from build123d import *

# Parameters (mm, degrees)
F0_R     = 2.1
F1_DEPTH = 6.16
F2_W     = 23
F2_H     = 3
F3_DEPTH = 12.5
F4_W     = 23
F4_H     = 20
F4_W_2   = 2.2
F4_H_2   = 1.7
F5_DEPTH = 1.6
F8_DEPTH = 2
F12_R    = 2


with BuildPart() as f1:
    # F0 (on Right) → F1 (new body)
    with BuildSketch(Plane.YZ):
        Polygon((-9.7124977037, -5.25), (9.7124977037, -5.25), (11.5, -3.4624977037), (11.5, 3.4624977037), (11.5, 5.25), (9.7124977037, 5.25), (-9.7124977037, 5.25), (-11.5, 5.25), (-11.5, 3.4624977037), (-11.5, -3.4624977037), align=None)
        with Locations((-6.35, 0)):
            Circle(F0_R, mode=Mode.SUBTRACT)
        with Locations((6.35, 0)):
            Circle(F0_R, mode=Mode.SUBTRACT)
    extrude(amount=F1_DEPTH)

    # F2 (on face) → F3 (join)
    with BuildSketch(Plane(origin=(0, 0, 0), x_dir=(0, -1, 0), z_dir=(-1, 0, 0))):
        with Locations((0, 6.75)):
            Rectangle(F2_W, F2_H)
    extrude(amount=-F3_DEPTH)

    # F4 (on face) → F5 (join)
    with BuildSketch(Plane.YZ.offset(12.5)):
        with Locations((0, 15.25)):
            Rectangle(F4_W, F4_H)
        with Locations((-2.65, 9.4)):
            Rectangle(F4_W_2, F4_H_2, mode=Mode.SUBTRACT)
        with Locations((2.65, 9.4)):
            Rectangle(F4_W_2, F4_H_2, mode=Mode.SUBTRACT)
        with Locations((-2.65, 23.1)):
            Rectangle(F4_W_2, F4_H_2, mode=Mode.SUBTRACT)
        with Locations((2.65, 23.1)):
            Rectangle(F4_W_2, F4_H_2, mode=Mode.SUBTRACT)
    extrude(amount=-F5_DEPTH)

    # F6: union 

    # F7 (on face) → F8 (join)
    with BuildSketch(Plane(origin=(0, 11.5, 0), x_dir=(-1, 0, 0), z_dir=(0, 1, 0))):
        Polygon((-5.45, 8.25), (-10.9, 14.6002341062), (-10.9, 8.25), align=None)
        Polygon((-6.16, 5.25), (-12.5, 5.25), (-6.16, -1.7691504909), align=None)
    extrude(amount=-F8_DEPTH)

    # F10: F1 across plane


with BuildPart() as f1_1:
    add(f1.part)
    add(f1.part.mirror(Plane.XZ))

    # F11: F1 across plane


with BuildPart() as f1_2:
    add(f1_1.part)
    add(f1_1.part.mirror(Plane.XZ))

    # F12
    f12_edges = [f1_2.edges().sort_by_distance(p)[0] for p in [
        (11.7, 11.5, 25.25),
        (11.7, -11.5, 25.25),
    ]]
    fillet(f12_edges, radius=F12_R)


solid = f1_2.part
The listing builds one solid part. Answer for the finished solid, in the listing's coordinates (mm). A direction names the side the tool comes from. Give positions to 0.01 mm unless a question says otherwise; leave off trailing zeros. Write each loop counter-clockwise with the first axis right and the second up, starting at its lowest first coordinate (ties: lowest second). Pieces come first, ordered by that corner, then holes.
Item 1: Section A-A, the plane y = -6.35 is taken. Write down the section's boundary in (x, z).
Item 2: Find the intervals of material crossed by line 1 along Y through (x, z) = (11.5, 23); line 2 along Y through (x, z) = (4.5, 0); line 3 along Z through (x, y) = (4.75, -6.35), in increasing order.
Item 3: Which of the six approach directions +Z, -Z, +X, -X, +Y, -Y give full straight-line access (tool end or side, diameter ignored) to faces 1 (the flat face through (3, 0, -5.25)), 2 (the flat face through (9, -9.5, 10)), 3 (the flat face through (12, 3, 8.55)), 4 (the flat face through (9, 0, 5.25))?
Item 4: Section D-D, the plane z = -1 is taken. Write down the section's boundary in (x, y).
Item 5: Determine the mould class of faces 5 (the flat face through (3.04, -10.62, -4.34)), 6 (the flat face through (9, 9.5, 10)), 7 (the flat face through (12, -1.55, 23)), 8 (the flat face through (8.137, 10.514, 11.381)) for opening direction Z: released by +Z, released by -Z, zero draft, split by the parting line, or undercut.
Item 6: Section C-C, the plane x = 4.25 is taken. Write down the section's boundary in (y, z), plus the area to 3 significant figures.
Item 7: Section B-B, the plane y = 3.25 is taken. Write down the section's boundary in (x, z).
Item 8: Flat-ended cylindrical pins translate along their axes: P1, Ø5, axis at y = -0.5, z = 1, coming from the +X side; P2, Ø0.8, axis at x = 11.5, y = -2, coming from the -Z side. Find the tip coordinate at first contact, or state that the pin passes through.
Completed:
1. outline: (0, -5.25) - (6.16, -5.25) - (6.16, -2.1) - (0, -2.1) - close; (0, 2.1) - (6.16, 2.1) - (6.16, 5.25) - (12.5, 5.25) - (12.5, 25.25) - (10.9, 25.25) - (10.9, 8.25) - (0, 8.25) - close
2. line 1: y = -11.5 to -3.75, -1.55 to 1.55, 3.75 to 11.5
2. line 2: y = -11.5 to -8.45, -4.25 to 4.25, 8.45 to 11.5
2. line 3: z = -5.25 to -2.1, 2.1 to 8.25
3. face 1: -Z, +X, -X, +Y, -Y
3. face 2: +Z, -X
3. face 3: +X, -X
3. face 4: -Z, +X
4. outline: (0, -11.5) - (6.85, -11.5) - (6.85, -9.5) - (6.16, -9.5) - (6.16, -8.2) - (0, -8.2) - close; (0, -4.5) - (6.16, -4.5) - (6.16, 4.5) - (0, 4.5) - close; (0, 8.2) - (6.16, 8.2) - (6.16, 9.5) - (6.85, 9.5) - (6.85, 11.5) - (0, 11.5) - close
5. face 5: released by -Z
5. face 6: zero draft
5. face 7: undercut
5. face 8: released by +Z
6. outline: (-11.5, -3.46) - (-9.71, -5.25) - (9.71, -5.25) - (11.5, -3.46) - (11.5, 8.25) - (-11.5, 8.25) - close; hole circle Ø4.2 at (-6.35, 0); hole circle Ø4.2 at (6.35, 0)
6. area: 280 mm2
7. outline: (0, -5.25) - (6.16, -5.25) - (6.16, 5.25) - (12.5, 5.25) - (12.5, 8.55) - (10.9, 8.55) - (10.9, 8.25) - (0, 8.25) - close; (10.9, 10.25) - (12.5, 10.25) - (12.5, 22.25) - (10.9, 22.25) - close; (10.9, 23.95) - (12.5, 23.95) - (12.5, 25.25) - (10.9, 25.25) - close
8. P1: stops at x = 6.16
8. P2: stops at z = 5.25
